Design review of the part built by this model. Coordinates are the model's own, in mm. Coordinates: 2 decimals unless noted, no trailing zeros. Loops run counter-clockwise (first coordinate to the right, second up) from the corner with the lowest first, then second, coordinate; pieces in that order, holes last. Notation, with made-up numbers: M 49,78.5 L 97,78.5 A21 cw 97,82.5 Z; hole C 43.25,52.25 d7. An arc over 180 degrees is marked long. Answer as CSV lines item,"result". Start each with the question number.
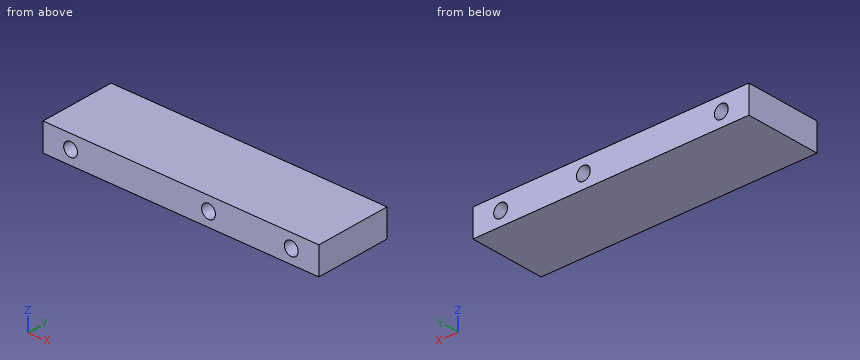
from build123d import *

# Parameters (mm, degrees)
F0_W     = 127
F0_H     = 12.7
F1_DEPTH = 34.925
F2_R     = 3.175
F3_DEPTH = 34.925


# Not quite as in the source:
# - a feature names something its author has since deleted; it is built from what else it names


with BuildPart() as f1:
    # F0 (on Front) → F1 (new body)
    with BuildSketch(Plane.XZ):
        with Locations((-31.0538060308, 35.6538111673)):
            Rectangle(F0_W, F0_H)
    extrude(amount=F1_DEPTH)

    # F2 (on face) → F3 (cut)
    with BuildSketch(Plane.XZ.offset(34.925)):
        with Locations((-81.8538060308, 35.6538111673)):
            Circle(F2_R)
        with Locations((-18.3538060308, 35.6538111673)):
            Circle(F2_R)
        with Locations((19.7461939692, 35.6538111673)):
            Circle(F2_R)
    extrude(amount=-F3_DEPTH, mode=Mode.SUBTRACT)


solid = f1.part
Item 1: Add section C-C (z = 34.5). Give the boundary of the cut face in (x, y) (3 decimals), plus the area to 3 significant figures.
Item 2: Add section B-B (y = -30.5). Give the boundary of the cut face in (x, z) (3 decimals), plus the area to 3 significant figures.
Item 3: Add section A-A (x = -81). Give the boundary of the cut face in (y, z) (3 decimals).
Item 4: For line 1 along X through (y, z) = (-22.5, 32.75); line 2 along X through (y, z) = (-16.5, 34); line 3 along Z through (x, y) = (-21, -33), list the stretches that pass through material, from the lowest coordinate up. Write a range as from..to.
Response:
1,outline,"M -94.554,-34.925 L -84.812,-34.925 L -84.812,0 L -94.554,0 Z; M -78.896,-34.925 L -21.312,-34.925 L -21.312,0 L -78.896,0 Z; M -15.396,-34.925 L 16.788,-34.925 L 16.788,0 L -15.396,0 Z; M 22.704,-34.925 L 32.446,-34.925 L 32.446,0 L 22.704,0 Z"
1,area,"3,820 mm²"
2,outline,"M -94.554,29.304 L 32.446,29.304 L 32.446,42.004 L -94.554,42.004 Z; hole C -81.854,35.654 d6.35; hole C -18.354,35.654 d6.35; hole C 19.746,35.654 d6.35"
2,area,"1,520 mm²"
3,outline,"M -34.925,29.304 L 0,29.304 L 0,32.596 L -34.925,32.596 Z; M -34.925,38.712 L 0,38.712 L 0,42.004 L -34.925,42.004 Z"
4,line 1,"-94.55..-83.14, -80.57..-19.64, -17.07..18.46, 21.03..32.45"
4,line 2,"-94.55..-84.56, -79.14..-21.06, -15.64..17.04, 22.46..32.45"
4,line 3,"29.3..33.9, 37.41..42"
